Verification items for this drawing (mm, ordinates from the low corner). A direction names the side the tool comes from. Coordinates: 2 decimals unless noted, no trailing zeros. Write each loop counter-clockwise with the first axis right and the second up, starting at its lowest first coordinate (ties: lowest second). Pieces come first, ordered by that corner, then holes. Notation, with made-up numbers: M 57,-21.75 L 114,-21.75 A18 cw 114,9.25 Z; hole C 42.5,69 d5. An arc over 180 degrees is marked long. Put each result on its own line as item: value. Start each with the question number.
1) Cross-section at C-C on z = 7. Record the cut outline in (x, y), plus the area to 3 significant figures.
2) Cross-section at D-D on z = 6. Record the cut outline in (x, y), plus the area to 3 significant figures.
3) Cross-section at A-A on x = 8.75. Record the cut outline in (y, z), plus the area to 3 significant figures.
4) Set-up check for the marked faces 1 and 2: record each of +Z, -Z, +X, -X, +Y, -Y from which the full face is reachable in a straight line by a thin tool's end or side.
5) Gauge pin test, flat end, axial feed: pin 1 (4 mm diameter, centred on x = 11.5, z = 6, fed in from +Y). Record the tip position at first contact, or that the pin passes through.
6) Scan lines: line 1 along Z through (x, y) = (4.5, 6); line 2 along Z through (x, y) = (10, 3.5); line 3 along X through (y, z) = (6.25, 1.75). Record each from-to range of solid material in increasing order.
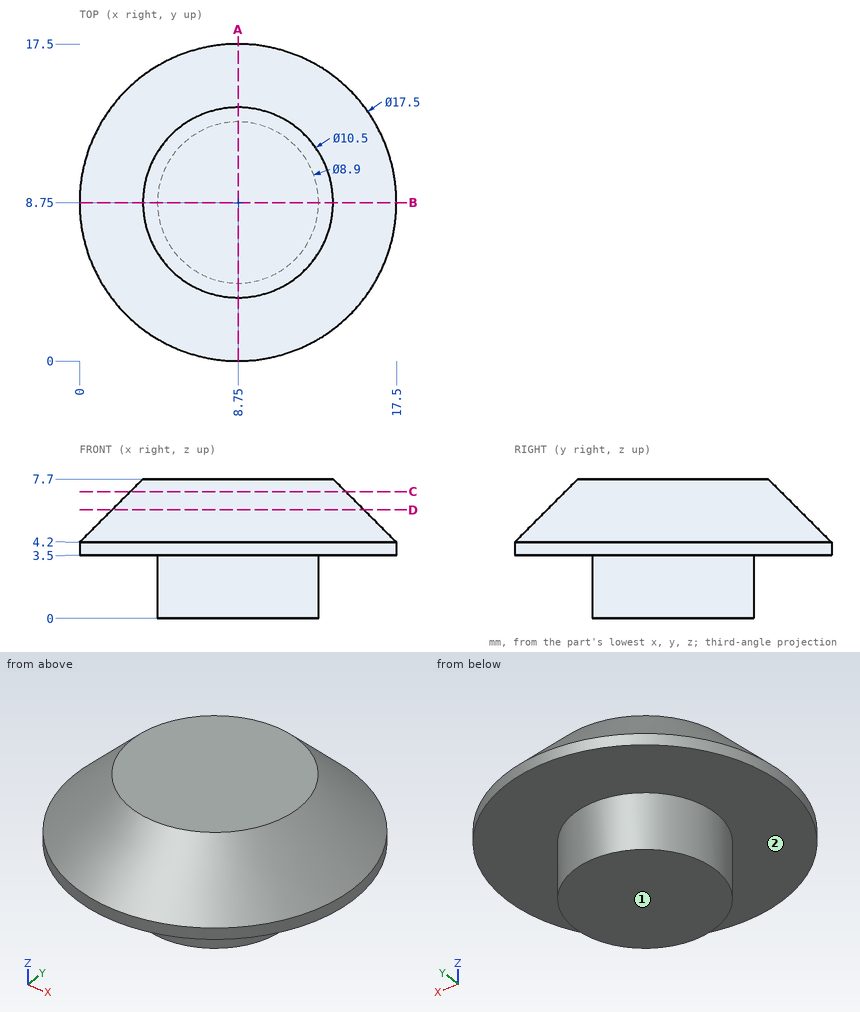
Answer key:
1. outline: C 8.75,8.75 d11.9
1. area: 111 mm²
2. outline: C 8.75,8.75 d13.9
2. area: 152 mm²
3. outline: M 0,3.5 L 4.3,3.5 L 4.3,0 L 13.2,0 L 13.2,3.5 L 17.5,3.5 L 17.5,4.2 L 14,7.7 L 3.5,7.7 L 0,4.2 Z
3. area: 92.4 mm²
4. face 1: -Z, +X, -X, +Y, -Y
4. face 2: -Z
5. pin 1: stops at y = 17.3
6. line 1: z = 3.5 to 7.7
6. line 2: z = 3.5 to 7.55
6. line 3: x = 5.07 to 12.43
